Design review of the part built by this model. Coordinates are the model's own, in mm. A direction names the side the tool comes from. Round coordinates to 2 decimals unless told otherwise and drop trailing zeros. Order: outer loops, then holes, each group sorted by start corner. A loop starts at its lowest first (then second) coordinate and runs counter-clockwise, first axis right, second up.
from build123d import *

# Parameters (mm, degrees)
F1_DEPTH = 1
F2_DEPTH = 4
F3_R     = 5


with BuildPart() as f1:
    # F0 (on Top) → F1 (new body)
    with BuildSketch(Plane.XY):
        Polygon((-15, 0), (0, 0), (15, 0), (15, 15), (0, 15), (0, 30), (-15, 30), align=None)
    extrude(amount=F1_DEPTH)

    # F0 (on Top) → F2 (join)
    with BuildSketch(Plane.XY):
        Polygon((15, 0), (0, 0), (-15, 0), (-15, 30), (-17, 30), (-17, -2), (0, -2), (15, -2), align=None)
        Polygon((0, 15), (15, 15), (15, 17), (2, 17), (2, 30), (0, 30), align=None)
    extrude(amount=F2_DEPTH)

    # F3
    f3_edges = [f1.edges().sort_by_distance(p)[0] for p in [
        (0, 15, 2.5),
        (-17, -2, 2),
        (2, 17, 2),
        (-15, 0, 2.5),
    ]]
    fillet(f3_edges, radius=F3_R)


solid = f1.part
1) Take a section at D-D on x = -2.5. Give the boundary of the cut face in (y, z).
Results:
outline: (-2, 0) - (30, 0) - (30, 1) - (0, 1) - (0, 4) - (-2, 4) - close
2) The part is to be moulded in two halves that separate along Y. For faces 1 (the face through (-5, 11, 0)), 2 (the face through (10, 15, 2)), 3 (the face through (11, 17, 2)), 4 (the face through (-4, 12, 1)), say which applies: released by +Y, released by -Y, zero draft, split by the parting line, or undercut.
Results:
face 1: zero draft
face 2: undercut
face 3: released by +Y
face 4: undercut
3) Clearance check with flat-ended pins moving along their axes: P1, Ø12, axis at x = -9, y = 5, coming from the -Z side; P2, Ø6, axis at x = 1, y = 10, coming from the +Z side; P3, Ø1.5, axis at x = -2.5, z = 3, coming from the +Y side; P4, Ø2, axis at y = 27, z = 2, coming from the +X side. State where each tip first meets the part, or that it passes through.
Results:
P1: stops at z = 0
P2: stops at z = 1
P3: stops at y = 0
P4: stops at x = 2
4) Take a section at A-A on x = 12. Give the boundary of the cut face in (y, z), plus the area to 3 significant figures.
Results:
outline: (-2, 0) - (17, 0) - (17, 4) - (15, 4) - (15, 1) - (0, 1) - (0, 4) - (-2, 4) - close
area: 31.0 mm2
5) For faces 5 (the face through (1, 17, 3)), 6 (the face through (2, 26, 2)), 7 (the face through (0, 25, 2)), list the 3-axis set-ups (+Z, -Z, +X, -X, +Y, -Y) from which the entire face can be reached by the end or side of a thin tool; tool diameter is ignored.
Results:
face 5: +Z
face 6: +Z, -Z, +X, +Y
face 7: +Z, +Y
6) Take a section at C-C on y = 18.5. Give the boundary of the cut face in (x, z), plus the area to 3 significant figures.
Results:
outline: (-17, 0) - (3.43, 0) - (3.43, 4) - (0.23, 4) - (0.23, 1) - (-15, 1) - (-15, 4) - (-17, 4) - close
area: 36.0 mm2
7) Take a section at B-B on z = 3.2. Give the boundary of the cut face in (x, y), plus the area to 3 significant figures.
Results:
outline: (-17, 3) arc R5 ccw to (-12, -2) - (15, -2) - (15, 0) - (-10, 0) arc R5 cw to (-15, 5) - (-15, 30) - (-17, 30) - close; (0, 20) arc R5 ccw to (5, 15) - (15, 15) - (15, 17) - (7, 17) arc R5 cw to (2, 22) - (2, 30) - (0, 30) - close
area: 180 mm2
8) To check wall thickness, follow line 1 along Y through (x, z) = (9, 2.3); line 2 along Y through (x, z) = (1, 2.35); line 3 along X through (y, z) = (28.5, 3.4). State the ranges of each line that lie inside material, in increasing order.
Results:
line 1: y = -2 to 0, 15 to 17
line 2: y = -2 to 0, 17 to 30
line 3: x = -17 to -15, 0 to 2
